Autodesk Inventor part; units mm, degrees
ref_plane "WorkPlane1" through (0, 0, 0) normal (0, 0, 1) x (1, 0, 0)
ref_plane "MSC_PF1" through (0, 0, 0) normal (1, 0, 0) x (0, 1, 0)
ref_plane "MSC_PT1" through (0, 0, 0) normal (0, 0, -1) x (-1, 0, 0)
ref_plane "WorkPlane1" through (0, 0, 0) normal (0, 0, 1) x (1, 0, 0)
sketch "Sketch1" plane through (0, 0, 0) normal (0, 0, 1) x (1, 0, 0)
  point P0 (0, 0)
sketch "Sketch2" plane through (0, 0, 0) normal (0, 0, 1) x (1, 0, 0)
  line L0 (-9, 5.1963) -> (-9, -5.1963)
  line L1 (0, 10.3922) -> (-9, 5.1963)
  line L2 (9, 5.1963) -> (0, 10.3922)
  line L3 (9, -5.1963) -> (9, 5.1963)
  line L4 (0, -10.3922) -> (9, -5.1963)
  line L5 (-9, -5.1963) -> (0, -10.3922)
  circle A0 centre (0, 0) radius 9 construction
  dimension "d1" = 18
  dimension "d29" = 0
  dimension "d30" = 0
extrude "Extrusion1" add sketch "Sketch2" along normal blind 7.5
sketch "Sketch3" plane through (0, 0, 0) normal (1, 0, 0) x (0, 1, 0)
  line L0 (9, 7.5) -> (10.4922, 7.5)
  line L1 (10.4922, 6.6385) -> (9, 7.5)
  line L2 (10.4922, 7.5) -> (10.4922, 6.6385)
  line L3 (0, -1.5) -> (0, 9)
  line L4 (10.3922, 0) -> (10.3922, 7.5)
  dimension "d25" = 0.1
  dimension "d26" = 0
  dimension "d27" = 60
  dimension "d28" = 9
revolve "Revolution1" cut sketch "Sketch3" angle 360 about axis through (0, 0, -10) along (0, 0, 1)
sketch "Sketch4" plane through (0, 0, 0) normal (1, 0, 0) x (0, 1, 0)
  line L0 (0, -70) -> (0, 0)
  line L1 (-6, -70) -> (0, -70)
  line L2 (-6, 0) -> (-6, -70)
  line L3 (0, 0) -> (-6, 0)
  line L4 (0, -70) -> (0, 0)
  line L5 (-7.2, 0) -> (1.2, 0)
  line L6 (0, -84) -> (0, 14)
  dimension "d18" = 6
  dimension "d20" = 70
  dimension "d33" = 0
  dimension "d34" = 0
revolve "Revolution2" add sketch "Sketch4" angle 360 about axis through (0, 0, -70) along (0, 0, -1)
chamfer "Chamfer1" distance 0.875 angle 45 1 edges at (0, 6, -70)
fillet "Fillet1" radius 0.6 1 edges at (0, 6, 0)
thread "Thread1"
ref_plane "MSC_PF1" through (0, 0, 0) normal (1, 0, 0) x (0, 1, 0)
ref_plane "MSC_PT1" through (0, 0, 0) normal (0, 0, -1) x (-1, 0, 0)
equation "\"d22\" = 0.5 * PTC"
equation "\"d23\" = 0.5 * PTC"
equation "\"d24\" = r"
equation "\"d1\" = ParS"
equation "\"d6\" = ParK"
equation "\"b\" = NLG - 2 * PTC"
equation "\"d28\" = 0.5 * ParS"
equation "\"d18\" = 0.5 * NND"
equation "\"d20\" = NLG"
equation "\"NND\" = 12"
equation "\"NLG\" = 70"
equation "\"PTC\" = 1.75"
equation "\"ParK\" = 7.5"
equation "\"ParS\" = 18"
equation "\"msp_es\" = 0.577367 * ParS"
equation "\"r\" = 0.6"
equation "\"THREADDIA\" = NND"
properties part number "ISO 4018 - M12 x 70" material "Steel"
Work out the finished part from the listing and answer in its coordinate system (mm). A direction names the side the tool comes from. Coordinates: 2 decimals unless noted, no trailing zeros. Loops run counter-clockwise (first coordinate to the right, second up) from the corner with the lowest first, then second, coordinate; pieces in that order, holes last. Notation, with made-up numbers: M 83,37.25 L 95,37.25 A23 cw 95,68.25 Z; hole C 3.25,-19 d1. An arc over 180 degrees is marked long. Answer in a Markdown table with one row per item. Add a question column.
1. Consider L1, parallel to Z at x = 6.75, y = 5; L2, parallel to X at y = -2, z = -58; L3, parallel to Y at x = 4.75, z = -24. Determine where each line is inside the solid, lowest interval first.
2. A tool of negligible diameter and unlimited length cuts with its end or side. For faces 1 (the cylindrical face through (0, 6, -35)), 2 (the flat face through (4.56, 7.76, 3.7)), from which of +Z, -Z, +X, -X, +Y, -Y can it reach the whole face along a straight path? Write none if from no direction.
3. Flat-ended cylindrical pins translate along their axes: P1, Ø2, axis at x = 6.5, y = -8, coming from the +Z side; P2, Ø1, axis at y = 5, z = -44, coming from the -X side; P3, Ø5, axis at x = -6, z = -40, coming from the -Y side; P4, Ø1, axis at x = 3.5, z = -17, coming from the -Y side. Find the tip coordinate at first contact, or state that the pin passes through.
4. Find section A-A, the plane z = -65. Write down the section's boundary in (x, y), then the cut area to 3 significant figures.
Reported:
| question | item | result |
|---|---|---|
| 1 | L1 | z = 0 to 7.5 |
| 1 | L2 | x = -5.66 to 5.66 |
| 1 | L3 | y = -3.67 to 3.67 |
| 2 | face 1 | -Z |
| 2 | face 2 | +Z, -Z, +X, +Y |
| 3 | P1 | passes through |
| 3 | P2 | stops at x = -3.97 |
| 3 | P3 | stops at y = -4.87 |
| 3 | P4 | stops at y = -5.2 |
| 4 | outline | C 0,0 d12 |
| 4 | area | 113 mm^2 |
